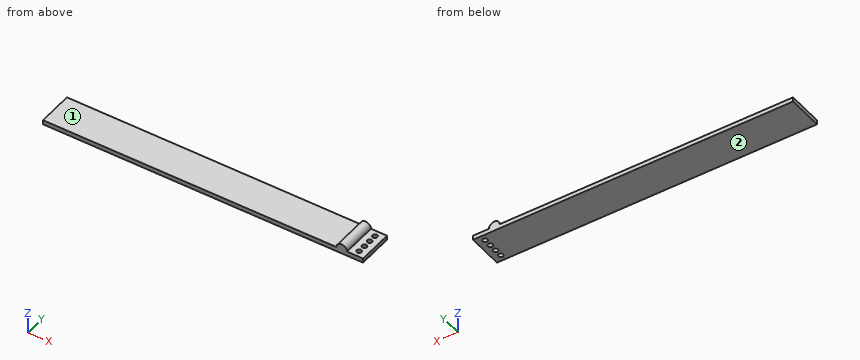
from build123d import *

# Parameters (mm, degrees)
F0_W     = 457.2
F0_H     = 50.8
F1_DEPTH = 6.35
F3_DEPTH = 50.8
F4_R     = 3.429
F5_DEPTH = 25.4


with BuildPart() as f1:
    # F0 (on Top) → F1 (new body)
    with BuildSketch(Plane.XY):
        Rectangle(F0_W, F0_H)
    extrude(amount=F1_DEPTH)

    # F2 (on face) → F3 (join)
    with BuildSketch(Plane.XZ.offset(25.4)):
        with BuildLine():
            Line((190.5, 6.35), (205.74, 6.35))
            ThreePointArc((205.74, 6.35), (198.12, 13.97), (190.5, 6.35))
        make_face()
    extrude(amount=-F3_DEPTH)

    # F4 (on face) → F5 (cut)
    with BuildSketch(Plane.XY.offset(6.35)):
        with Locations((217.17, -16.764)):
            Circle(F4_R)
        with Locations((217.17, -5.588)):
            Circle(F4_R)
        with Locations((217.17, 5.588)):
            Circle(F4_R)
        with Locations((217.17, 16.764)):
            Circle(F4_R)
    extrude(amount=-F5_DEPTH, mode=Mode.SUBTRACT)


solid = f1.part
Read the model definition and answer for the solid it produces. Units are mm, in the model's axes. Face numbers are marked on the shaded views. A direction names the side the tool comes from. Coordinates: 2 decimals unless noted, no trailing zeros. Loops run counter-clockwise (first coordinate to the right, second up) from the corner with the lowest first, then second, coordinate; pieces in that order, holes last.
Q1. Consider probe 1 along Y at (x, z) = (217.17, 2.5) (3 decimals); probe 2 along X at (y, z) = (-1.5, 7.5); probe 3 along Z at (x, y) = (83, 3). Determine where each line is inside the solid, lowest interval first.
Q2. Each of these flat-tipped pins is pushed along its axis until it touches: pin 1 Ø5.5 at (x, y) = (217.17, -16.764) entering from -Z (3 decimals); pin 2 Ø8 at (x, y) = (217.17, 16.764) entering from +Z. Where does it stop, or does it pass through?
Q3. The part is cut by section B-B on z = 10.25. Write down the section's boundary in (x, y), and give its area (3 significant figures).
Q4. The part is cut by section A-A on x = -148.5. Write down the section's boundary in (y, z).
Q5. Which of the six approach directions +Z, -Z, +X, -X, +Y, -Y give full straight-line access (tool end or side, diameter ignored) to the marked faces 1 and 2?
Results below:
1. probe 1: y = -25.4 to -20.193, -13.335 to -9.017, -2.159 to 2.159, 9.017 to 13.335, 20.193 to 25.4
1. probe 2: x = 190.59 to 205.65
1. probe 3: z = 0 to 6.35
2. pin 1: passes through
2. pin 2: stops at z = 6.35
3. outline: (191.57, -25.4) - (204.67, -25.4) - (204.67, 25.4) - (191.57, 25.4) - close
3. area: 665 mm2
4. outline: (-25.4, 0) - (25.4, 0) - (25.4, 6.35) - (-25.4, 6.35) - close
5. face 1: +Z, -X, +Y, -Y
5. face 2: -Z, +X, -X, +Y, -Y
